Job drawing, mm, ordinate dimensions from the low corner. One solid piece. Give positions to 0.01 mm unless a question says otherwise; leave off trailing zeros. Loops run counter-clockwise (first coordinate to the right, second up) from the corner with the lowest first, then second, coordinate; pieces in that order, holes last. Notation, with made-up numbers: M 70.25,59 L 75.25,59 A8 cw 75.25,72 Z; hole C -2.75,-21 d11. An arc over 180 degrees is marked long. One line per question, with ' | ' between items.
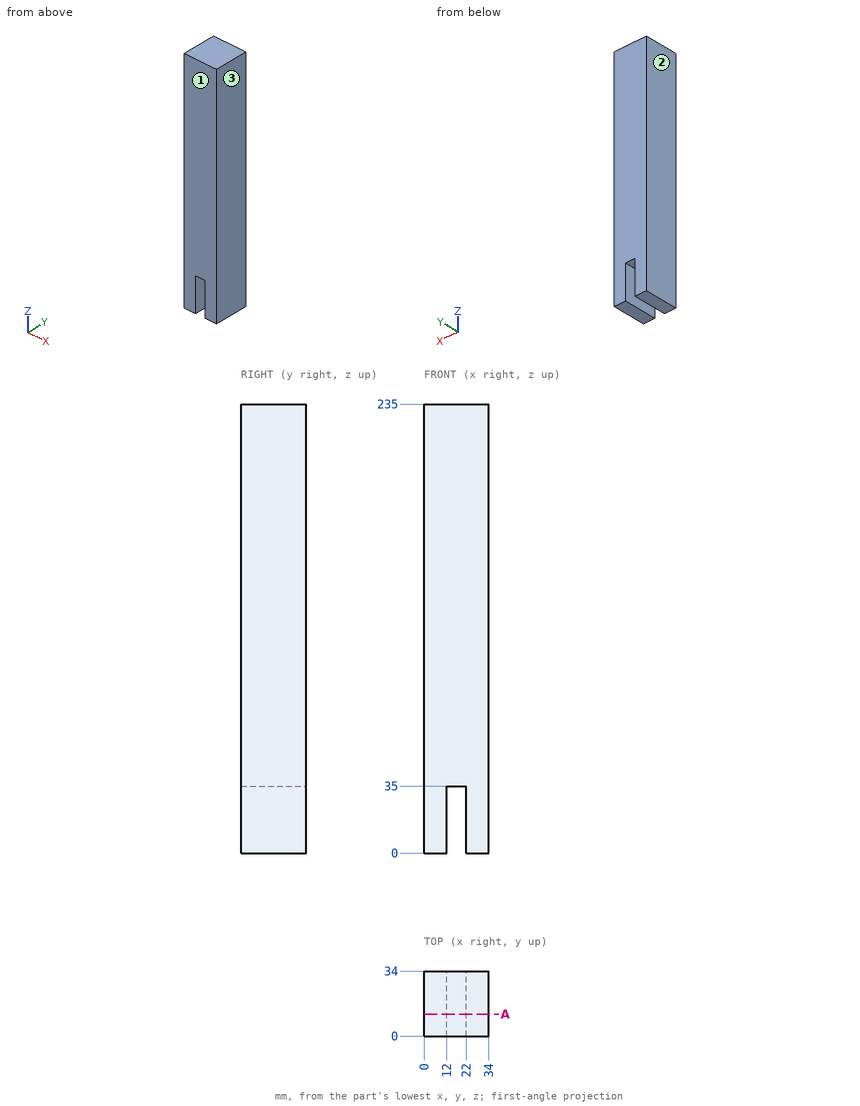
Item 1: Saw through at A-A on y = 11.5. Give the cut face in (x, z).
Conclusion:
outline: M 0,0 L 12,0 L 12,35 L 22,35 L 22,0 L 34,0 L 34,235 L 0,235 Z
Item 2: Mould opens along X. For the marked faces 1, 2 and 3 say: pulls with the +X half, pulls with the -X half, needs draft (parallel to the pull), parting line crosses it, or undercut.
Conclusion:
face 1: needs draft | face 2: pulls with the -X half | face 3: pulls with the +X half
Item 3: Drop a flat-ended pin along its axis: P1, Ø5, axis at x = 18, y = 24.5, coming from the -Z side. Give the stop position or say it passes through.
Conclusion:
P1: z = 35
Item 4: Drill centre lines: line 1 along X through (y, z) = (2.5, 34.5); line 2 along Z through (x, y) = (18, 18.5). Where is each one in solid material? Low to high. Write a range as [from, to].
Conclusion:
line 1: [0, 12], [22, 34] | line 2: [35, 235]
